For this review, take the finished solid that the model builds, in its own axes (mm). A direction names the side the tool comes from. Round coordinates to 2 decimals unless told otherwise and drop trailing zeros. Loops run counter-clockwise (first coordinate to the right, second up) from the corner with the lowest first, then second, coordinate; pieces in that order, holes last.
1) Insertion check: pin 1 (1.5 mm diameter, centred on x = 4, z = 17.5, fed in from +Y); pin 2 (1.5 mm diameter, centred on y = -17, z = -13, fed in from +X); pin 3 (1 mm diameter, centred on x = 2, z = 1.5, fed in from +Y). Each pin has a flat end and moves straight along its axis. Give the tip position at first contact, or say it passes through.
2) Mouldability with a two-part tool opening along Z and no side actions: class faces 4 (the flat face through (0, -6, 0)), 5 (the conical face through (8.437, -25.718, -5.711)), 6 (the flat face through (8.708, -4, -2)) as pulls with the +Z half, pulls with the -Z half, needs draft (parallel to the pull), parting line crosses it, or undercut.
3) Take a section at C-C (x = 6.5). State the section outline as (y, z) points.
4) Tool access review of faces 1 (the conical face through (8.351, -24.973, -5.545)), 2 (the cylindrical face through (5.188, -2.03, 4.896)), 3 (the cylindrical face through (4.842, 4.065, -0.534)): name each direction out of +Z, -Z, +X, -X, +Y, -Y from which nothing blocks a thin tool from reaching the whole face with its end or side.
5) Take a section at A-A (z = 0). State the section outline as (x, y) points.
6) Wall thickness on L1, parallel to X at y = 4, z = 19.5; L2, parallel to Y at x = 1.75, z = 2; L3, parallel to Z at x = 1.5, y = 20.5: over which ranges is each line inside the solid? List them lowest first.
```python
from build123d import *

# Parameters (mm, degrees)
F2_SIZE2 = 0.8660254038
F2_SIZE  = 0.5
F3_SIZE2 = 0.8660254038
F3_SIZE  = 0.5
F4_SIZE  = 0.5


with BuildPart() as f1:
    # F0 (on Front) → F1 (revolve)
    with BuildSketch(Plane.XZ):
        Polygon((0, 4.1), (8.7081384471, 4.1), (8.7081384471, 5.3), (0.9, 5.3), (0.9, 28.81), (8.7081384471, 25.4264733396), (9, 26.1), (0, 30), align=None)
    revolve(axis=Axis((3.0769170262, 0, 0), (-1, 0, 0)))

    # F2
    f2_edges = [f1.edges().sort_by_distance(p)[0] for p in [
        (0, 0, -4.1),
    ]]
    f2_side = f1.faces().sort_by_distance((0, 0, -29.151472))[0]
    chamfer(f2_edges, length=F2_SIZE, length2=F2_SIZE2, reference=f2_side)

    # F3
    f3_edges = [f1.edges().sort_by_distance(p)[0] for p in [
        (0.9, 0, -5.3),
    ]]
    f3_side = f1.faces().sort_by_distance((0.9, 0, -6.11487))[0]
    chamfer(f3_edges, length=F3_SIZE, length2=F3_SIZE2, reference=f3_side)

    # F4
    f4_edges = [f1.edges().sort_by_distance(p)[0] for p in [
        (0.9, 0, -28.81),
    ]]
    chamfer(f4_edges, length=F4_SIZE)


solid = f1.part
```
Response:
1. pin 1: stops at y = 22.9
1. pin 2: stops at x = 0.9
1. pin 3: stops at y = 29.31
2. face 4: needs draft
2. face 5: parting line crosses it
2. face 6: undercut
3. outline: circle Ø54.37 at (0, 0); circle Ø10.6 at (0, 0); hole circle Ø52.77 at (0, 0); hole circle Ø8.2 at (0, 0)
4. face 1: none
4. face 2: +X
4. face 3: +X, -X
5. outline: (0, -30) - (9, -26.1) - (8.71, -25.43) - (1.36, -28.61) - (0.9, -28.31) - (0.9, -5.8) - (1.77, -5.3) - (8.71, -5.3) - (8.71, -4.1) - (0.87, -4.1) - (0, -4.6) - close; (0, 4.6) - (0.87, 4.1) - (8.71, 4.1) - (8.71, 5.3) - (1.77, 5.3) - (0.9, 5.8) - (0.9, 28.31) - (1.36, 28.61) - (8.71, 25.43) - (9, 26.1) - (0, 30) - close
6. L1: x = 0 to 0.9
6. L2: y = -29.17 to -28.37, -4.92 to -3.58, 3.58 to 4.92, 28.37 to 29.17
6. L3: z = -21 to -19.87, 19.87 to 21
